Part model, mm, in its own coordinate system. A direction names the side the tool comes from. Round coordinates to 2 decimals unless told otherwise and drop trailing zeros. Loops run counter-clockwise (first coordinate to the right, second up) from the corner with the lowest first, then second, coordinate; pieces in that order, holes last.
1) Band-saw the part on C-C, the plane z = 7.5. Write the cut outline in (x, y), then the cut area to 3 significant figures.
2) 3-axis set-ups, long thin cutter, end or side, ignore diameter. For faces 1 (the flat face through (44, -10, 137)), 2 (the flat face through (30, -1, 21)), 3 (the flat face through (20, -1, 77)), 4 (the flat face through (44, -18, 8)), 5 (the cylindrical face through (15, -5, 142)): which of +Z, -Z, +X, -X, +Y, -Y reach the whole face in a straight line?
3) Band-saw the part on B-B, the plane x = 42.5. State how many separate pieces and enclosed holes the cut face has, then the cut area to 3 significant figures.
4) Probe line 1 (Z direction, x = 15, y = -4); line 2 (X direction, y = -5.5, z = 144.5); line 3 (Z direction, x = 53.5, y = -10). List the from-to ranges inside material, lowest first.
5) Drop flat-ended pins along their axis: P1, Ø0.9, axis at y = -2, z = 22.5, coming from the +X side; P2, Ø2.5, axis at y = -1, z = 130, coming from the -X side; P3, Ø5, axis at x = 24, z = 78.5, coming from the -Y side. Give the stop position or say it passes through.
6) Band-saw the part on A-A, the plane y = -5.25. Write the cut outline in (x, z), then the cut area to 3 significant figures.
7) Mould opens along Z. For faces 6 (the flat face through (44, -9, 0)), 7 (the flat face through (0, -9, 145)), 8 (the flat face through (30, -1, 131)), 9 (the flat face through (45, -1, 117)) say: +Z half, -Z half, draft (parallel to the pull), parting line (faces both ways), or undercut.
from build123d import *

# Parameters (mm, degrees)
PAD_DEPTH    = 3
SKETCH001_W  = 90
SKETCH001_H  = 15
PAD001_DEPTH = 15
SKETCH002_R  = 2.5
POCKET_DEPTH = 10


with BuildPart() as part:
    # Sketch → Pad (new body)
    with BuildSketch(Plane.XZ):
        Polygon((0, 152), (0, 137), (20, 137.000045), (20, 15), (0, 15), (0, 0), (90, 0), (90, 15), (70, 15), (70, 137.000045), (90, 137.000045), (90, 152), align=None)
        with BuildLine():
            ThreePointArc((30, 124.5), (32.196699, 119.196699), (37.5, 117))
            Line((37.5, 117), (52.5, 117))
            ThreePointArc((52.5, 117), (57.803301, 119.196699), (60, 124.5))
            Line((60, 124.5), (60, 137))
            Line((60, 137), (30, 137))
            Line((30, 124.5), (30, 137))
        make_face(mode=Mode.SUBTRACT)
        with BuildLine():
            ThreePointArc((37.5, 35), (32.196699, 32.803301), (30, 27.5))
            Line((30, 27.5), (30, 15))
            Line((30, 15), (60, 15))
            Line((60, 15), (60, 27.5))
            ThreePointArc((60, 27.5), (57.803301, 32.803301), (52.5, 35))
            Line((52.5, 35), (37.5, 35))
        make_face(mode=Mode.SUBTRACT)
    extrude(amount=PAD_DEPTH)

    # Sketch001 (on Face26 of Pad) → Pad001 (join)
    with BuildSketch(Plane.XZ.offset(3)):
        Polygon((0, 152), (0, 137), (90, 137.000045), (90, 152), align=None)
        with Locations((45, 7.5)):
            Rectangle(SKETCH001_W, SKETCH001_H)
    extrude(amount=PAD001_DEPTH)

    # Sketch002 (on Face2 of Pad001) → Pocket (cut)
    with BuildSketch(Plane(origin=(0, 0, 0), x_dir=(1, 0, 0), z_dir=(0, 1, 0))):
        with Locations((15, -7.5)):
            Circle(SKETCH002_R)
        with Locations((75, -7.5)):
            Circle(SKETCH002_R)
        with Locations((75, -144.5)):
            Circle(SKETCH002_R)
        with Locations((15, -144.5)):
            Circle(SKETCH002_R)
    extrude(amount=-POCKET_DEPTH, mode=Mode.SUBTRACT)


solid = part.part
Reported:
1. outline: (0, -18) - (90, -18) - (90, 0) - (77.5, 0) - (77.5, -10) - (72.5, -10) - (72.5, 0) - (17.5, 0) - (17.5, -10) - (12.5, -10) - (12.5, 0) - (0, 0) - close
1. area: 1,520 mm2
2. face 1: +X, -X, -Y
2. face 2: +Y, -Y
2. face 3: -X, +Y, -Y
2. face 4: +Z, -Z, +X, -X, -Y
2. face 5: +Y
3. separate pieces: 3
3. enclosed holes: 0
3. area: 786 mm2
4. line 1: z = 0 to 5, 10 to 15, 137 to 142, 147 to 152
4. line 2: x = 0 to 12.5, 17.5 to 72.5, 77.5 to 90
4. line 3: z = 0 to 15, 137 to 152
5. P1: stops at x = 70
5. P2: stops at x = 20
5. P3: stops at y = -3
6. outline: (0, 0) - (90, 0) - (90, 15) - (0, 15) - close; (0, 137) - (90, 137) - (90, 152) - (0, 152) - close; hole circle Ø5 at (15, 7.5); hole circle Ø5 at (15, 144.5); hole circle Ø5 at (75, 7.5); hole circle Ø5 at (75, 144.5)
6. area: 2,620 mm2
7. face 6: -Z half
7. face 7: draft
7. face 8: undercut
7. face 9: undercut
